```python
from build123d import *


with BuildPart() as part:
    # Sketch1 → Revolve1 (revolve)
    with BuildSketch(Plane(origin=(0, 0, 0), x_dir=(0, 0, -1), z_dir=(1, 0, 0)), mode=Mode.PRIVATE) as revolve1_sk:
        with BuildLine():
            Line((0, 30.5), (0, 33.65))
            ThreePointArc((0, 33.65), (0.058578644, 33.791421356), (0.2, 33.85))
            Line((0.2, 33.85), (4.135594176, 33.85))
            ThreePointArc((4.135594176, 33.85), (4.497341053, 33.871889996), (4.853808838, 33.937240535))
            Line((4.853808838, 33.937240535), (8.15, 34.75))
            Line((8.15, 34.75), (8.15, 33.5))
            Line((8.15, 33.5), (4.91, 32.555))
            ThreePointArc((4.91, 32.555), (4.55005161, 32.0678162), (4.923849273, 31.591175658))
            Line((4.923849273, 31.591175658), (8.15, 30.75))
            Line((8.15, 30.75), (8.15, 29.3))
            Line((8.15, 29.3), (4.889181759, 30.193374861))
            ThreePointArc((4.889181759, 30.193374861), (4.496398447, 30.273224225), (4.096476318, 30.3))
            Line((4.096476318, 30.3), (0.2, 30.3))
            ThreePointArc((0.2, 30.3), (0.058578644, 30.358578644), (0, 30.5))
        make_face()
    revolve(revolve1_sk.sketch.rotate(Axis((0, 0, 0), (0, 0, -1)), 90), axis=Axis((0, 0, 0), (0, 0, -1)))


solid = part.part
```
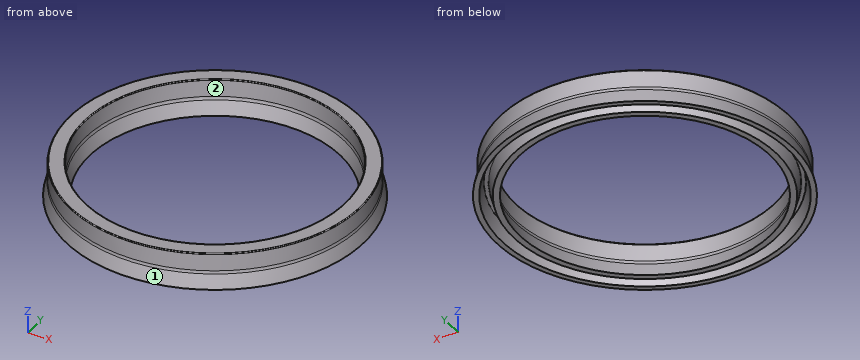
Can you work these out from the model? Positions are in its coordinate system, mm. Face numbers are marked on the shaded views. Round coordinates to 2 decimals unless told otherwise and drop trailing zeros. Order: outer loops, then holes, each group sorted by start corner. A loop starts at its lowest first (then second) coordinate and runs counter-clockwise, first axis right, second up.
(1) I'm going to push flat-ended pins straight in: pin 1 (3 mm diameter, centred on y = 9.5, z = -1.5, fed in from +X); pin 2 (1 mm diameter, centred on y = 4, z = -3.5, fed in from -X); pin 3 (4 mm diameter, centred on y = -23.5, z = -6, fed in from +X). Where does each tip first touch, or does it pass through?
Results are:
pin 1: stops at x = 32.89
pin 2: stops at x = -33.67
pin 3: stops at x = 26.74
(2) If we section it at C-C (z = -6.75): Please give me the cut outline in (x, y).
Results are:
outline: circle Ø68.81 at (0, 0); circle Ø62.23 at (0, 0); hole circle Ø66.18 at (0, 0); hole circle Ø59.37 at (0, 0)
(3) If we section it at A-A (x = 0): Please give me the cut outline in (y, z) (3 decimals).
Results are:
outline: (-34.75, -8.15) - (-33.5, -8.15) - (-32.555, -4.91) arc R0.5 cw to (-31.591, -4.924) - (-30.75, -8.15) - (-29.3, -8.15) - (-30.193, -4.889) arc R3 cw to (-30.3, -4.096) - (-30.3, -0.2) arc R0.2 ccw to (-30.5, 0) - (-33.65, 0) arc R0.2 ccw to (-33.85, -0.2) - (-33.85, -4.136) arc R3 cw to (-33.937, -4.854) - close; (29.3, -8.15) - (30.75, -8.15) - (31.591, -4.924) arc R0.5 cw to (32.555, -4.91) - (33.5, -8.15) - (34.75, -8.15) - (33.937, -4.854) arc R3 cw to (33.85, -4.136) - (33.85, -0.2) arc R0.2 ccw to (33.65, 0) - (30.5, 0) arc R0.2 ccw to (30.3, -0.2) - (30.3, -4.096) arc R3 cw to (30.193, -4.889) - close
(4) If I drill on L1, parallel to Y at x = 0, z = -2.9; L2, parallel to X at y = 12, z = -7.25; L3, parallel to X at y = 25.5, z = -6.5, over which ranges is the centre line in solid material (lowest first)?
Results are:
L1: y = -33.85 to -30.3, 30.3 to 33.85
L2: x = -32.38 to -31, -28.57 to -27, 27 to 28.57, 31 to 32.38
L3: x = -23 to -20.98, -17.94 to -15.33, 15.33 to 17.94, 20.98 to 23
(5) We'd pull the mould along Y, two halves only. Please class the marked faces 1 and 2: +Y half, -Y half, draft (parallel to the pull), parting line (faces both ways), or undercut.
Results are:
face 1: parting line
face 2: undercut
